from build123d import *

# Parameters (mm, degrees)
EXTRUDE_1_DEPTH     = 1
SKETCH_2_W          = 50
SKETCH_2_H          = 55
CUT_EXTRUDE_1_DEPTH = 1


with BuildPart() as part:
    # 草图1 → 凸台-拉伸1 (new body)
    with BuildSketch(Plane(origin=(0, 0, 0), x_dir=(0, 0, -1), z_dir=(1, 0, 0))):
        Polygon((0, 0), (0, 60), (32.139380484, 98.302222156), (92.139380484, 98.302222156), (124.278760969, 60), (124.278760969, 0), align=None)
    extrude(amount=-EXTRUDE_1_DEPTH)

    # 草图2 → 切除-拉伸1 (cut)
    with BuildSketch(Plane(origin=(0, 0, 0), x_dir=(0, 0, -1), z_dir=(1, 0, 0))):
        with Locations((50, 27.5)):
            Rectangle(SKETCH_2_W, SKETCH_2_H)
    extrude(amount=-CUT_EXTRUDE_1_DEPTH, mode=Mode.SUBTRACT)


solid = part.part
Source: CAD feature listing. Evaluate the final solid. Frame: model axes, mm. Coordinates: 2 decimals unless noted, no trailing zeros. Loops run counter-clockwise (first coordinate to the right, second up) from the corner with the lowest first, then second, coordinate; pieces in that order, holes last. Notation, with made-up numbers: (84, 85.25) - (142, 85.25) arc R23 cw to (142, 96.25) - close; hole circle Ø7 at (28.5, 15.5). An arc over 180 degrees is marked (long way). One line per question, with ' | ' between items.
1) Section C-C, the plane z = -73.5. Return loops of the section in (x, y).
Report:
outline: (-1, 55) - (0, 55) - (0, 98.3) - (-1, 98.3) - close
2) Section B-B, the plane x = -0.2. Return loops of the section in (y, z), then the cut area to 3 significant figures.
Report:
outline: (0, -124.28) - (60, -124.28) - (98.3, -92.14) - (98.3, -32.14) - (60, 0) - (0, 0) - (0, -25) - (55, -25) - (55, -75) - (0, -75) - close | area: 8,240 mm²
3) Section D-D, the plane y = 74. Return loops of the section in (x, z), then the cut area to 3 significant figures.
Report:
outline: (-1, -112.53) - (0, -112.53) - (0, -11.75) - (-1, -11.75) - close | area: 101 mm²
4) Line query: line 1 along Z through (x, y) = (-0.35, 25.5); line 2 along Y through (x, z) = (-0.5, -39.5); line 3 along Y through (x, z) = (-0.7, -96). Output: solid intervals per line, ascending.
Report:
line 1: z = -124.28 to -75, -25 to 0 | line 2: y = 55 to 98.3 | line 3: y = 0 to 93.7
5) Section A-A, the plane y = 18. Return loops of the section in (x, z), then the cut area to 3 significant figures.
Report:
outline: (-1, -124.28) - (0, -124.28) - (0, -75) - (-1, -75) - close; (-1, -25) - (0, -25) - (0, 0) - (-1, 0) - close | area: 74.3 mm²
6) First-contact query: P1, Ø0.5, axis at x = -0.5, z = -41, coming from the -Y side. Flat tip, straight axial feed; report the tip coordinate or a pass-through.
Report:
P1: stops at y = 55
